Source: three-view drawing plus pictorial views. Frame: mm from the lowest corner of the part. A direction names the side the tool comes from. Coordinates: 2 decimals unless noted, no trailing zeros. Write each loop counter-clockwise with the first axis right and the second up, starting at its lowest first coordinate (ties: lowest second). Pieces come first, ordered by that corner, then holes. Notation, with made-up numbers: M -19,54.25 L 24,54.25 A31 ccw 24,81.25 Z; hole C 47,55 d2. An arc over 180 degrees is marked long. Write item = value, one per line. Start each with the question number.
Item 1: Section D-D on x = 29. Output: boundary loops of the cut face in (y, z), plus the area to 3 significant figures.
Item 2: Section C-C on z = 105. Output: boundary loops of the cut face in (x, y).
Item 3: Reachability of the marked faces 4, 5 and 6 from +Z, -Z, +X, -X, +Y, -Y: full face, straight path, thin tool, end or side. Return the list, or none.
Item 4: Section A-A on x = 68.58. Output: boundary loops of the cut face in (y, z), plus the area to 3 significant figures.
Item 5: Section B-B on y = 50.8. Output: boundary loops of the cut face in (x, z).
Item 6: Ray query, L1, parallel to X at y = 20, z = 165; L2, parallel to Z at x = 52, y = 50.5; L3, parallel to Z at x = 109, y = 42. Return the intervals inside material, ascending. Write a range as [from, to].
Item 7: Pull-direction query (Z, two-part tool) for the marked faces 1, 2 and 3; classes: +Z half, -Z half, draft (parallel to the pull), parting line (faces both ways), or undercut.
Item 8: First-contact query: pin 1 Ø1.5 at (y, z) = (60.5, 73.5) entering from -X; pin 2 Ø3 at (x, y) = (89, 84) entering from -Z; pin 3 Ø2 at (x, z) = (71.5, 39) entering from -Y. Flat tips, straight axial feed; report the tip coordinate or a pass-through.
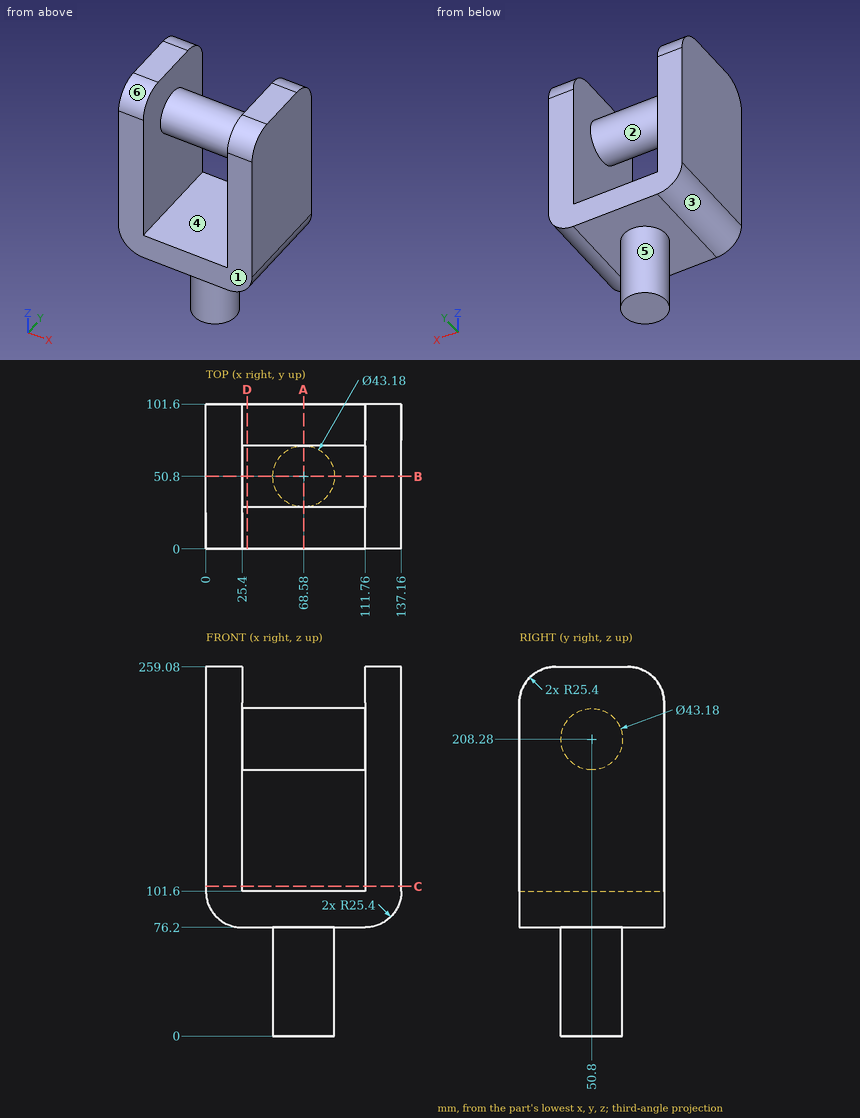
Responses:
q1.outline = M 0,76.2 L 101.6,76.2 L 101.6,101.6 L 0,101.6 Z; C 50.8,208.28 d43.18
q1.area = 4,050 mm²
q2.outline = M 0,0 L 25.4,0 L 25.4,101.6 L 0,101.6 Z; M 111.76,0 L 137.16,0 L 137.16,101.6 L 111.76,101.6 Z
q3.face_4 = +Y, -Y
q3.face_5 = -Z
q3.face_6 = +Z, +X, -X, -Y
q4.outline = M 0,76.2 L 29.21,76.2 L 29.21,0 L 72.39,0 L 72.39,76.2 L 101.6,76.2 L 101.6,101.6 L 0,101.6 Z; C 50.8,208.28 d43.18
q4.area = 7,340 mm²
q5.outline = M 0,101.6 A25.4 ccw 25.4,76.2 L 46.99,76.2 L 46.99,0 L 90.17,0 L 90.17,76.2 L 111.76,76.2 A25.4 ccw 137.16,101.6 L 137.16,259.08 L 111.76,259.08 L 111.76,229.87 L 25.4,229.87 L 25.4,259.08 L 0,259.08 Z; hole M 25.4,101.6 L 111.76,101.6 L 111.76,186.69 L 25.4,186.69 Z
q6.L1 = [0, 25.4], [111.76, 137.16]
q6.L2 = [0, 101.6], [186.69, 229.87]
q6.L3 = [76.2, 101.6], [188.56, 228]
q7.face_1 = draft
q7.face_2 = undercut
q7.face_3 = -Z half
q8.pin_1 = 48.93
q8.pin_2 = 76.2
q8.pin_3 = 29.3
